For this review, take the finished solid that the model builds, in its own axes (mm). A direction names the side the tool comes from. Coordinates: 2 decimals unless noted, no trailing zeros. Loops run counter-clockwise (first coordinate to the right, second up) from the corner with the lowest first, then second, coordinate; pieces in that order, holes last.
1. Machinability: for faces 5 (the face through (8.31, -23.678, -13.545)), 6 (the face through (-7.25, -0.45, 2.09)), 7 (the face through (-19.895, -0.449, 2.194)), which of the approach directions +Z, -Z, +X, -X, +Y, -Y give a long, thin tool a straight path to every point of the face, cutting with its end or side? Answer none if there is none.
2. Take a section at D-D, the plane y = 24.5. State the section outline as (x, z) points.
3. Take a section at C-C, the plane y = 65. State the section outline as (x, z) points, then the cut area to 3 significant figures.
4. To check wall thickness, follow probe 1 along X at (y, z) = (-13, -10); probe 2 along X at (y, z) = (-17, -10.21); probe 3 along Y at (x, z) = (9, -22.5). State the ranges of each line that lie inside material, in increasing order.
5. Clearance check with flat-ended pins moving along their axes: P1, Ø3.5, axis at x = 14.5, y = -18.5, coming from the +Z side; P2, Ø1.5, axis at x = 8.5, y = 18.5, coming from the -Z side; P3, Ø4, axis at x = 15.5, y = -18, coming from the -Z side; P4, Ø2, axis at x = 14.5, y = 49.5, coming from the -Z side. State where each tip first meets the part, or that it passes through.
6. Take a section at B-B, the plane y = -34. Count the separate pieces of the cut face and the enclosed holes in it, then the cut area to 3 significant figures.
7. Mouldability with a two-part tool opening along X and no side actions: class faces 1 (the face through (20.47, -0.45, 2.09)), 2 (the face through (-19.36, -23.68, -6.79)), 3 (the face through (-7.67, -23.68, 9.12)), 4 (the face through (-11.107, 3.972, -26.789)) as pulls with the +X half, pulls with the -X half, needs draft (parallel to the pull), parting line crosses it, or undercut.
8. Take a section at A-A, the plane x = 0. State the section outline as (y, z) points, then the cut area to 3 significant figures.
```python
from build123d import *

# Parameters (mm, degrees)
SKETCH1_W                 = 91.997104186
SKETCH1_H                 = 68.052652412
BOSS_EXTRUDE1_DEPTH       = 8
SKETCH2_R                 = 16
BOSS_EXTRUDE2_DEPTH       = 36
SKETCH3_R                 = 12.5
BOSS_EXTRUDE3_DEPTH       = 35
FILLET1_R                 = 0.5
FILLET2_R                 = 0.5
CHAMFER1_SIZE             = 3
CHAMFER2_SIZE             = 3
BOSS_EXTRUDE4_DEPTH       = 48
CHAMFER3_SIZE             = 1
CHAMFER4_SIZE             = 1
FILLET4_R                 = 1
SKETCH7_OUTSIDE_W         = 128.188
SKETCH7_OUTSIDE_H         = 104.242
SKETCH7_OUTSIDE_R         = 29
CUT_EXTRUDE1_DEPTH        = 40
CHAMFER5_SIZE             = 2
F_4_0MM_DOWEL_HOLE1_D     = 4
F_4_0MM_DOWEL_HOLE1_DEPTH = 48
F_4_0MM_DOWEL_HOLE1_TIP   = 1.201721238


with BuildPart() as part:
    # Sketch1 → Boss-Extrude1 (new body)
    with BuildSketch(Plane(origin=(0, 0, 0), x_dir=(1, 0, 0), z_dir=(0, 1, 0))):
        Rectangle(SKETCH1_W, SKETCH1_H)
    extrude(amount=BOSS_EXTRUDE1_DEPTH)

    # Sketch2 → Boss-Extrude2 (add)
    with BuildSketch(Plane(origin=(0, 8, 0), x_dir=(1, 0, 0), z_dir=(0, 1, 0))):
        with Locations(Location((0, 0, 0), (0, 0, 270))):
            Circle(SKETCH2_R)
    extrude(amount=BOSS_EXTRUDE2_DEPTH)

    # Sketch3 → Boss-Extrude3 (add)
    with BuildSketch(Plane(origin=(0, 44, 0), x_dir=(1, 0, 0), z_dir=(0, 1, 0))):
        with Locations(Location((0, 0, 0), (0, 0, 270))):
            Circle(SKETCH3_R)
    extrude(amount=BOSS_EXTRUDE3_DEPTH)

    # Fillet1
    fillet1_edges = [part.edges().sort_by_distance(p)[0] for p in [
        (0, 44, -12.5),
    ]]
    fillet(fillet1_edges, radius=FILLET1_R)

    # Fillet2
    fillet2_edges = [part.edges().sort_by_distance(p)[0] for p in [
        (0, 44, -16),
    ]]
    fillet(fillet2_edges, radius=FILLET2_R)

    # Chamfer1
    chamfer1_edges = [part.edges().sort_by_distance(p)[0] for p in [
        (0, 79, -12.5),
    ]]
    chamfer(chamfer1_edges, length=CHAMFER1_SIZE)

    # Chamfer2
    chamfer2_edges = [part.edges().sort_by_distance(p)[0] for p in [
        (0, 8, -16),
    ]]
    chamfer(chamfer2_edges, length=CHAMFER2_SIZE)

    # Sketch4 → Boss-Extrude4 (add)
    with BuildSketch(Plane.XZ):
        Polygon((6.384573519, -10.21), (10.281687836, -16.96), (18.075916471, -16.96), (21.973030788, -10.21), (18.075916471, -3.46), (10.281687836, -3.46), align=None)
        Polygon((6.384573519, 5.79), (10.281687836, -0.96), (18.075916471, -0.96), (21.973030788, 5.79), (18.075916471, 12.54), (10.281687836, 12.54), align=None)
        Polygon((-21.335426481, 5.79), (-17.438312164, -0.96), (-9.644083529, -0.96), (-5.746969212, 5.79), (-9.644083529, 12.54), (-17.438312164, 12.54), align=None)
        Polygon((-21.335426481, -10.21), (-17.438312164, -16.96), (-9.644083529, -16.96), (-5.746969212, -10.21), (-9.644083529, -3.46), (-17.438312164, -3.46), align=None)
    extrude(amount=BOSS_EXTRUDE4_DEPTH)

    # Chamfer3
    chamfer3_edges = [part.edges().sort_by_distance(p)[0] for p in [
        (8.333130678, 0, -13.585),
        (14.178802154, 0, -16.96),
        (20.024473629, 0, -13.585),
        (20.024473629, 0, -6.835),
        (14.178802154, 0, -3.46),
        (8.333130678, 0, -6.835),
        (0, 0, 34.026326206),
        (-45.998552093, 0, 0),
        (8.333130678, 0, 2.415),
        (0, 0, -34.026326206),
        (14.178802154, 0, -0.96),
        (20.024473629, 0, 2.415),
        (20.024473629, 0, 9.165),
        (14.178802154, 0, 12.54),
        (8.333130678, 0, 9.165),
        (45.998552093, 0, 0),
        (-19.386869322, 0, 2.415),
        (-13.541197846, 0, -0.96),
        (-7.695526371, 0, 2.415),
        (-7.695526371, 0, 9.165),
        (-13.541197846, 0, 12.54),
        (-19.386869322, 0, 9.165),
        (-19.386869322, 0, -13.585),
        (-13.541197846, 0, -16.96),
        (-7.695526371, 0, -13.585),
        (-7.695526371, 0, -6.835),
        (-13.541197846, 0, -3.46),
        (-19.386869322, 0, -6.835),
    ]]
    chamfer(chamfer3_edges, length=CHAMFER3_SIZE)

    # Chamfer4
    chamfer4_edges = [part.edges().sort_by_distance(p)[0] for p in [
        (8.333130678, -48, -13.585),
        (14.178802154, -48, -16.96),
        (20.024473629, -48, -13.585),
        (20.024473629, -48, -6.835),
        (14.178802154, -48, -3.46),
        (8.333130678, -48, -6.835),
        (8.333130678, -48, 2.415),
        (14.178802154, -48, -0.96),
        (20.024473629, -48, 2.415),
        (20.024473629, -48, 9.165),
        (14.178802154, -48, 12.54),
        (8.333130678, -48, 9.165),
        (-19.386869322, -48, 2.415),
        (-13.541197846, -48, -0.96),
        (-7.695526371, -48, 2.415),
        (-7.695526371, -48, 9.165),
        (-13.541197846, -48, 12.54),
        (-19.386869322, -48, 9.165),
        (-19.386869322, -48, -13.585),
        (-13.541197846, -48, -16.96),
        (-7.695526371, -48, -13.585),
        (-7.695526371, -48, -6.835),
        (-13.541197846, -48, -3.46),
        (-19.386869322, -48, -6.835),
    ]]
    chamfer(chamfer4_edges, length=CHAMFER4_SIZE)

    # Fillet4
    fillet4_edges = [part.edges().sort_by_distance(p)[0] for p in [
        (10.281687836, -24, 12.54),
        (6.384573519, -24, 5.79),
        (18.075916471, -24, 12.54),
        (21.973030788, -24, 5.79),
        (18.075916471, -24, -0.96),
        (10.281687836, -24, -0.96),
        (-17.438312164, -24, 12.54),
        (-21.335426481, -24, 5.79),
        (-9.644083529, -24, 12.54),
        (-5.746969212, -24, 5.79),
        (-9.644083529, -24, -0.96),
        (-17.438312164, -24, -0.96),
        (-17.438312164, -24, -3.46),
        (-21.335426481, -24, -10.21),
        (-9.644083529, -24, -3.46),
        (-5.746969212, -24, -10.21),
        (-9.644083529, -24, -16.96),
        (-17.438312164, -24, -16.96),
        (10.281687836, -24, -3.46),
        (6.384573519, -24, -10.21),
        (18.075916471, -24, -3.46),
        (21.973030788, -24, -10.21),
        (18.075916471, -24, -16.96),
        (10.281687836, -24, -16.96),
    ]]
    fillet(fillet4_edges, radius=FILLET4_R)

    # Sketch7 outside → Cut-Extrude1 (cut)
    with BuildSketch(Plane.XZ):
        Rectangle(SKETCH7_OUTSIDE_W, SKETCH7_OUTSIDE_H)
        with Locations(Location((0, 0, 0), (0, 0, 270))):
            Circle(SKETCH7_OUTSIDE_R, mode=Mode.SUBTRACT)
    extrude(amount=-CUT_EXTRUDE1_DEPTH, mode=Mode.SUBTRACT)

    # Chamfer5
    chamfer5_edges = [part.edges().sort_by_distance(p)[0] for p in [
        (0, 8, 29),
        (0, 0, 29),
    ]]
    chamfer(chamfer5_edges, length=CHAMFER5_SIZE)

    # Ø4.0mm Dowel Hole1
    with Locations(Plane.XZ.offset(48)):
        with Locations((14.178802154, 5.79), (-13.541197846, 5.79), (-13.541197846, -10.21), (14.178802154, -10.21)):
            Hole(F_4_0MM_DOWEL_HOLE1_D / 2, depth=F_4_0MM_DOWEL_HOLE1_DEPTH)
            with Locations((0, 0, -(F_4_0MM_DOWEL_HOLE1_DEPTH + F_4_0MM_DOWEL_HOLE1_TIP / 2))):  # 118° drill point
                Cone(0, F_4_0MM_DOWEL_HOLE1_D / 2, F_4_0MM_DOWEL_HOLE1_TIP, mode=Mode.SUBTRACT)


solid = part.part
```
Results list:
1. face 5: -Z, -Y
1. face 6: -Y
1. face 7: -X, -Y
2. outline: circle Ø32 at (0, 0)
3. outline: circle Ø25 at (0, 0)
3. area: 491 mm2
4. probe 1: x = -21.16 to -15.53, -11.55 to -5.92, 6.56 to 12.19, 16.17 to 21.8
4. probe 2: x = -21.18 to -15.54, -11.54 to -5.9, 6.54 to 12.18, 16.18 to 21.82
4. probe 3: y = 0 to 8
5. P1: stops at z = 12.54
5. P2: stops at z = -14
5. P3: stops at z = -16.96
5. P4: passes through
6. separate pieces: 4
6. enclosed holes: 4
6. area: 580 mm2
7. face 1: pulls with the +X half
7. face 2: pulls with the -X half
7. face 3: undercut
7. face 4: parting line crosses it
8. outline: (0, -27) - (2, -29) - (6, -29) - (8, -27) - (8, -19) - (11, -16) - (43.5, -16) arc R0.5 ccw to (44, -15.5) - (44, -13) arc R0.5 cw to (44.5, -12.5) - (76, -12.5) - (79, -9.5) - (79, 9.5) - (76, 12.5) - (44.5, 12.5) arc R0.5 cw to (44, 13) - (44, 15.5) arc R0.5 ccw to (43.5, 16) - (11, 16) - (8, 19) - (8, 27) - (6, 29) - (2, 29) - (0, 27) - close
8. area: 2,480 mm2
